Geometry check sheet. Reference: the model listing, model coordinates, mm. Face numbers are marked on the shaded views. Coordinates: 2 decimals unless noted, no trailing zeros. Loops run counter-clockwise (first coordinate to the right, second up) from the corner with the lowest first, then second, coordinate; pieces in that order, holes last.
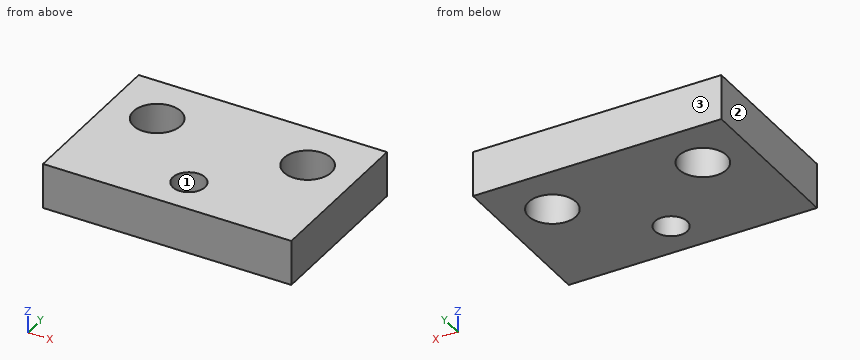
from build123d import *

# Parameters (mm, degrees)
SKETCH_1_W          = 33
SKETCH_1_H          = 22
EXTRUDE_1_DEPTH     = 6
SKETCH_2_R          = 3.15
SKETCH_2_R_2        = 2.15
CUT_EXTRUDE_1_DEPTH = 6


with BuildPart() as part:
    # 草图1 → 凸台-拉伸1 (new body)
    with BuildSketch(Plane.XY):
        with Locations((0, 11)):
            Rectangle(SKETCH_1_W, SKETCH_1_H)
    extrude(amount=EXTRUDE_1_DEPTH)

    # 草图2 → 切除-拉伸1 (cut)
    with BuildSketch(Plane.XY):
        with Locations((-10, 15)):
            Circle(SKETCH_2_R)
        with Locations((0, 5)):
            Circle(SKETCH_2_R_2)
        with Locations(Location((10, 15, 0), (0, 0, 180))):
            Circle(SKETCH_2_R)
    extrude(amount=CUT_EXTRUDE_1_DEPTH, mode=Mode.SUBTRACT)


solid = part.part
1) Mould release check, pull along X, two halves, no side actions. Record for the marked faces 1, 2 and 3: +X half, -X half, draft (parallel to the pull), parting line (faces both ways), or undercut.
Data:
face 1: undercut
face 2: -X half
face 3: draft
2) Depth check by flat-ended pin: pin 1 (4 mm diameter, centred on x = -10, y = 15, fed in from +Z); pin 2 (1.5 mm diameter, centred on x = -11, z = 4, fed in from -Y). Enter the tip coordinate at first touch or a pass-through.
Data:
pin 1: passes through
pin 2: stops at y = 0
3) Section check C-C on z = 0.4. Record the cut outline in (x, y), and give its area (3 significant figures).
Data:
outline: (-16.5, 0) - (16.5, 0) - (16.5, 22) - (-16.5, 22) - close; hole circle Ø6.3 at (-10, 15); hole circle Ø4.3 at (0, 5); hole circle Ø6.3 at (10, 15)
area: 649 mm2
4) Section check B-B on y = 15. Record the cut outline in (x, z), and give its area (3 significant figures).
Data:
outline: (-16.5, 0) - (-13.15, 0) - (-13.15, 6) - (-16.5, 6) - close; (-6.85, 0) - (6.85, 0) - (6.85, 6) - (-6.85, 6) - close; (13.15, 0) - (16.5, 0) - (16.5, 6) - (13.15, 6) - close
area: 122 mm2
5) Section check A-A on x = 10. Record the cut outline in (y, z).
Data:
outline: (0, 0) - (11.85, 0) - (11.85, 6) - (0, 6) - close; (18.15, 0) - (22, 0) - (22, 6) - (18.15, 6) - close
6) Material ranges on probe 1 along Y at (x, z) = (-10, 2.8); probe 2 along X at (y, z) = (17.25, 2.5); probe 3 along Y at (x, z) = (0, 4.05), recorded low to high.
Data:
probe 1: y = 0 to 11.85, 18.15 to 22
probe 2: x = -16.5 to -12.2, -7.8 to 7.8, 12.2 to 16.5
probe 3: y = 0 to 2.85, 7.15 to 22
7) Section check D-D on y = 5. Record the cut outline in (x, z).
Data:
outline: (-16.5, 0) - (-2.15, 0) - (-2.15, 6) - (-16.5, 6) - close; (2.15, 0) - (16.5, 0) - (16.5, 6) - (2.15, 6) - close
